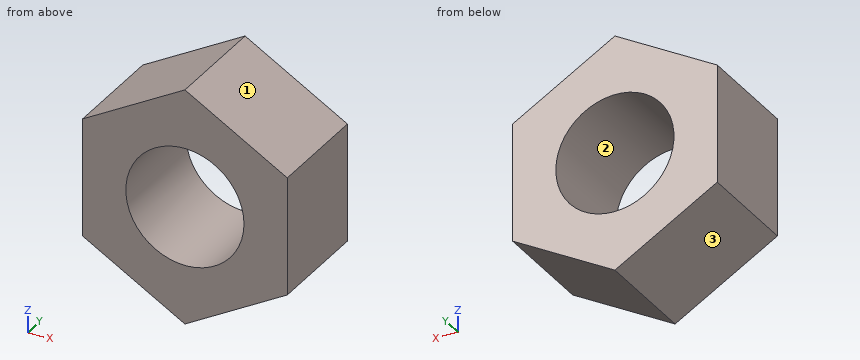
Solid Edge part; units mm, degrees
sketch "Sketch1" plane through (0, 0, 0) normal (0, -1, 0) x (1, 0, 0)
  line L0 (5.5, 3.1754) -> (0, 6.3509)
  line L1 (0, 6.3509) -> (-5.5, 3.1754)
  line L2 (-5.5, 3.1754) -> (-5.5, -3.1754)
  line L3 (-5.5, -3.1754) -> (0, -6.3509)
  line L4 (0, -6.3509) -> (5.5, -3.1754)
  line L5 (5.5, -3.1754) -> (5.5, 3.1754)
  circle A0 centre (0, 0) radius 3.175
extrude "Protrusion1" add sketch "Sketch1" against normal blind 5.7
Source: CAD feature listing. Evaluate the final solid. Frame: model axes, mm. Face numbers are marked on the shaded views. Give positions to 0.01 mm unless a question says otherwise; leave off trailing zeros. Write each loop counter-clockwise with the first axis right and the second up, starting at its lowest first coordinate (ties: lowest second). Pieces come first, ordered by that corner, then holes. Notation, with made-up numbers: M -37.75,43.5 L 9.25,43.5 A19 ccw 9.25,78.5 Z; hole C 27,76.25 d11. An arc over 180 degrees is marked long. Return JSON: item names as keys, results as strings. Group by question number.
1) Pin query (flat end, axial travel): P1, Ø2, axis at x = 2, y = 2, coming from the -Z side; P2, Ø2, axis at x = -4, y = 4.5, coming from the -Z side. Return the tip coordinate at first contact, or that it passes through.
2) Material intervals for line 1 along X through (y, z) = (3.45, -2.5); line 2 along Z through (x, y) = (1.75, 2.3); line 3 along Z through (x, y) = (-0.25, 3.6), sorted ascending. Write a range as [from, to].
3) Pull-direction query (Z, two-part tool) for the marked faces 1, 2 and 3; classes: pulls with the +Z half, pulls with the -Z half, needs draft (parallel to the pull), parting line crosses it, or undercut.
4) Cut plane D-D, the plane x = 4.25. Output: boundary loops of the cut face in (y, z).
5) Cut plane A-A, the plane z = 0. Output: boundary loops of the cut face in (x, y) (3 decimals).
6) Cut plane B-B, the plane y = 1.9. Output: boundary loops of the cut face in (x, z) (3 decimals), plus the area to 3 significant figures.
7) Cut plane C-C, the plane x = 1.25. Output: boundary loops of the cut face in (y, z), plus the area to 3 significant figures.
Recorded:
{
 "1": {"P1": "stops at z = -5.77", "P2": "stops at z = -4.62"},
 "2": {"line 1": "x = [-5.5, -1.96], [1.96, 5.5]", "line 2": "z = [-5.34, -2.65], [2.65, 5.34]", "line 3": "z = [-6.21, -3.17], [3.17, 6.21]"},
 "3": {"face 1": "pulls with the +Z half", "face 2": "undercut", "face 3": "pulls with the -Z half"},
 "4": {"outline": "M 0,-3.9 L 5.7,-3.9 L 5.7,3.9 L 0,3.9 Z"},
 "5": {"outline": "M -5.5,0 L -3.175,0 L -3.175,5.7 L -5.5,5.7 Z; M 3.175,0 L 5.5,0 L 5.5,5.7 L 3.175,5.7 Z"},
 "6": {"outline": "M -5.5,-3.175 L 0,-6.351 L 5.5,-3.175 L 5.5,3.175 L 0,6.351 L -5.5,3.175 Z; hole C 0,0 d6.35", "area": "73.1 mm²"},
 "7": {"outline": "M 0,-5.63 L 5.7,-5.63 L 5.7,-2.92 L 0,-2.92 Z; M 0,2.92 L 5.7,2.92 L 5.7,5.63 L 0,5.63 Z", "area": "30.9 mm²"}
}
